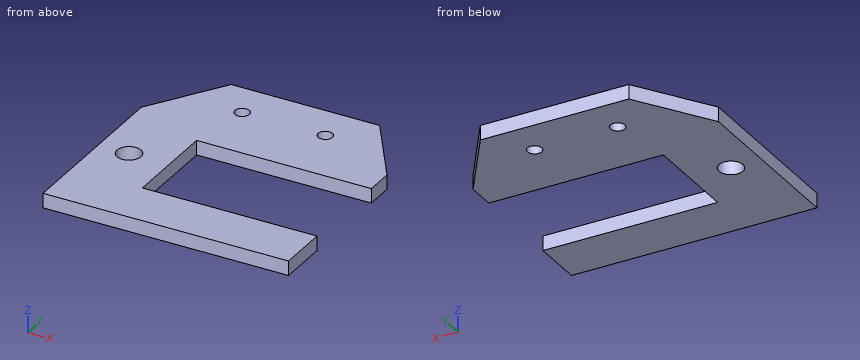
```python
from build123d import *

# Parameters (mm, degrees)
SKETCH1_R           = 2.5
SKETCH1_R_2         = 1.5
SKETCH1_W           = 25.402305243
SKETCH1_H           = 10.51
BOSS_EXTRUDE1_DEPTH = 3


with BuildPart() as part:
    # Sketch1 → Boss-Extrude1 (new body)
    # profile 1 of 3: a face of its own
    with BuildSketch(Plane.XY):
        Polygon((-25.402305243, -12.3212841), (0, -12.3212841), (0, -1.8112841), (-10.737694757, -1.8112841), (-10.737694757, 18.1887159), (0, 18.1887159), (0, 39.160695464), (-15.365, 39.160695464), (-25.402305243, 23.9787159), align=None)
        with Locations((-19.052305243, 8.0787159)):
            Circle(SKETCH1_R, mode=Mode.SUBTRACT)
        with Locations((-8.602305243, 31.190695464)):
            Circle(SKETCH1_R_2, mode=Mode.SUBTRACT)
    # profile 2 of 3: a face of its own
    with BuildSketch(Plane.XY):
        Polygon((0, 39.160695464), (0, 18.1887159), (25.402305243, 18.1887159), (25.402305243, 23.9787159), (15.365, 39.160695464), align=None)
        with Locations((8.602305243, 31.190695464)):
            Circle(SKETCH1_R_2, mode=Mode.SUBTRACT)
    # profile 3 of 3: a face of its own
    with BuildSketch(Plane.XY):
        with Locations((12.701152622, -7.0662841)):
            Rectangle(SKETCH1_W, SKETCH1_H)
    extrude(amount=BOSS_EXTRUDE1_DEPTH)


solid = part.part
```
Model file for the job. Use its own axes, mm. Coordinates: 2 decimals unless noted, no trailing zeros. Loops run counter-clockwise (first coordinate to the right, second up) from the corner with the lowest first, then second, coordinate; pieces in that order, holes last. Notation, with made-up numbers: M 56.25,15 L 106.25,15 A18 cw 106.25,38 Z; hole C 67.25,17.5 d1. An arc over 180 degrees is marked long. Use CSV: the item, a comma, the result in double quotes. Start each with the question number.
1. Probe probe 1 along Y at (x, z) = (-2.5, 1.6); probe 2 along X at (y, z) = (32.5, 0.2); probe 3 along X at (y, z) = (31.5, 2.35). List the from-to ranges inside material, lowest first. Write a range as [from, to].
2. Band-saw the part on D-D, the plane y = 34. List the corners of the cut face in (x, z), then the cut area to 3 significant figures.
3. Band-saw the part on A-A, the plane x = -4. List the corners of the cut face in (y, z), then the cut area to 3 significant figures.
4. Flat gauge pin, fed straight in: pin 1 (2.5 mm diameter, centred on x = -8.6, y = 31.19, fed in from +Z). Where does the tip first touch, or does it go through?
5. Band-saw the part on B-B, the plane y = 9. List the corners of the cut face in (x, z).
6. Band-saw the part on C-C, the plane z = 0.55. List the corners of the cut face in (x, y) (3 decimals), then the cut area to 3 significant figures.
Entries:
1,probe 1,"y = [-12.32, -1.81], [18.19, 39.16]"
1,probe 2,"x = [-19.77, -9.33], [-7.87, 7.87], [9.33, 19.77]"
1,probe 3,"x = [-20.43, -10.07], [-7.13, 7.13], [10.07, 20.43]"
2,outline,"M -18.78,0 L 18.78,0 L 18.78,3 L -18.78,3 Z"
2,area,"113 mm2"
3,outline,"M -12.32,0 L -1.81,0 L -1.81,3 L -12.32,3 Z; M 18.19,0 L 39.16,0 L 39.16,3 L 18.19,3 Z"
3,area,"94.4 mm2"
4,pin 1,"passes through"
5,outline,"M -25.4,0 L -21.38,0 L -21.38,3 L -25.4,3 Z; M -16.73,0 L -10.74,0 L -10.74,3 L -16.73,3 Z"
6,outline,"M -25.402,-12.321 L 25.402,-12.321 L 25.402,-1.811 L -10.738,-1.811 L -10.738,18.189 L 25.402,18.189 L 25.402,23.979 L 15.365,39.161 L -15.365,39.161 L -25.402,23.979 Z; hole C -19.052,8.079 d5; hole C -8.602,31.191 d3; hole C 8.602,31.191 d3"
6,area,"1,710 mm2"
